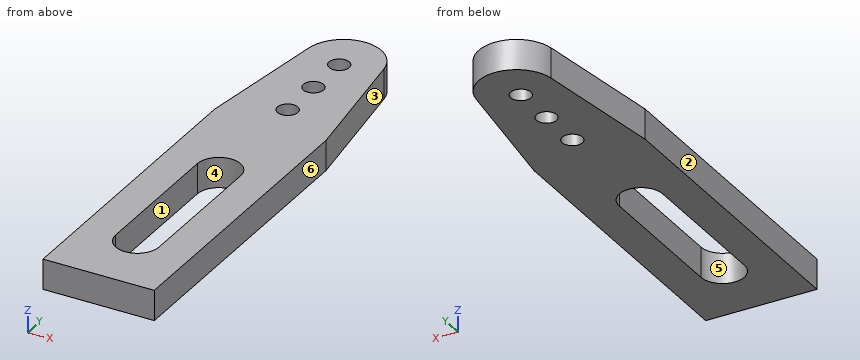
Autodesk Inventor part; units mm, degrees
ref_plane "YZ Plane" through (0, 0, 0) normal (1, 0, 0) x (0, 1, 0)
ref_plane "XZ Plane" through (0, 0, 0) normal (0, 1, 0) x (-1, 0, 0)
ref_plane "XY Plane" through (0, 0, 0) normal (0, 0, 1) x (1, 0, 0)
sketch "Sketch1" plane through (0, 0, 0) normal (0, 0, 1) x (1, 0, 0)
  line L0 (0, 0) -> (7.35, 0)
  line L1 (7.35, 0) -> (7.35, 20)
  line L2 (7.35, 20) -> (0, 20)
  line L3 (0, 20) -> (0, 0)
  circle A0 centre (3.68, 28.5) radius 2.5
  line L4 (1.2028, 28.8372) -> (0, 20)
  line L5 (6.1575, 28.8344) -> (7.35, 20)
  circle A1 centre (3.68, 28) radius 0.67
  circle A2 centre (3.68, 4.5) radius 1.43
  circle A3 centre (3.68, 14) radius 1.43
  circle A4 centre (3.68, 25) radius 0.67
  circle A5 centre (3.68, 22) radius 0.67
  line L6 (2.25, 4.5) -> (2.25, 14)
  line L7 (5.11, 14) -> (5.11, 4.5)
  point P0 (5.11, 4.5)
  dimension "d0" = 7.35
  dimension "d1" = 20
  dimension "d2" = 5
  dimension "d3" = 28.5
  dimension "d4" = 3.68
  dimension "d5" = 1.34
  dimension "d6" = 2.86
  dimension "d7" = 2.86
  dimension "d8" = 1.34
  dimension "d9" = 1.34
  dimension "d10" = 28
  dimension "d11" = 3.68
  dimension "d12" = 25
  dimension "d13" = 3.68
  dimension "d14" = 3.68
  dimension "d15" = 22
  dimension "d16" = 14
  dimension "d17" = 4.5
  dimension "d18" = 3.68
  dimension "d19" = 3.68
extrude "Extrusion1" add sketch "Sketch1" along normal blind 2
properties part number "Standard Servo Horn - Linear Arm"
Verification items for the finished model (mm, model axes). Face numbers are marked on the shaded views. A direction names the side the tool comes from. Give positions to 0.01 mm unless a question says otherwise; leave off trailing zeros. Write each loop counter-clockwise with the first axis right and the second up, starting at its lowest first coordinate (ties: lowest second). Pieces come first, ordered by that corner, then holes. Notation, with made-up numbers: M 88,43.25 L 92,43.25 A7 cw 92,50.25 Z; hole C -0.75,42 d5. An arc over 180 degrees is marked long. Write item = value, one per line.
(1) Access from +Z, -Z, +X, -X, +Y, -Y to the whole of each face (thin tool, end or side, straight path). Record for the marked faces 5 and 6.
Found:
face_5 = +Z, -Z
face_6 = +Z, -Z, +X, +Y, -Y
(2) Sectioned sample at D-D (y = 28). Record the cut outline in (x, z), then the cut area to 3 significant figures.
Found:
outline = M 1.09,0 L 3.01,0 L 3.01,2 L 1.09,2 Z; M 4.35,0 L 6.27,0 L 6.27,2 L 4.35,2 Z
area = 7.68 mm2
(3) Sectioned sample at C-C (z = 1). Record the cut outline in (x, y), then the cut area to 3 significant figures.
Found:
outline = M 0,0 L 7.35,0 L 7.35,20 L 6.16,28.83 A2.5 ccw 1.2,28.84 L 0,20 Z; hole M 2.25,4.5 A1.43 ccw 5.11,4.5 L 5.11,14 A1.43 ccw 2.25,14 Z; hole C 3.68,22 d1.34; hole C 3.68,25 d1.34; hole C 3.68,28 d1.34
area = 172 mm2
(4) Draft check along Y on the marked faces 1, 2, 3 and 4. Enter one of: released by +Y, released by -Y, zero draft, split by the parting line, or undercut.
Found:
face_1 = undercut
face_2 = zero draft
face_3 = released by +Y
face_4 = undercut
(5) Sectioned sample at B-B (x = 3.68). Record the cut outline in (y, z).
Found:
outline = M 0,0 L 3.07,0 L 3.07,2 L 0,2 Z; M 15.43,0 L 21.33,0 L 21.33,2 L 15.43,2 Z; M 22.67,0 L 24.33,0 L 24.33,2 L 22.67,2 Z; M 25.67,0 L 27.33,0 L 27.33,2 L 25.67,2 Z; M 28.67,0 L 31,0 L 31,2 L 28.67,2 Z
(6) Sectioned sample at A-A (y = 8). Record the cut outline in (x, z).
Found:
outline = M 0,0 L 2.25,0 L 2.25,2 L 0,2 Z; M 5.11,0 L 7.35,0 L 7.35,2 L 5.11,2 Z
(7) Material ranges on line 1 (Y direction, x = 3.68, z = 0.75); line 2 (X direction, y = 13, z = 1.9); line 3 (Y direction, x = 4.25, z = 1.2), recorded low to high.
Found:
line_1 = 0 to 3.07, 15.43 to 21.33, 22.67 to 24.33, 25.67 to 27.33, 28.67 to 31
line_2 = 0 to 2.25, 5.11 to 7.35
line_3 = 0 to 3.19, 15.31 to 21.65, 22.35 to 24.65, 25.35 to 27.65, 28.35 to 30.93
(8) Go/stop test with a flat-tipped pin: pin 1 Ø0.8 at (x, y) = (3.68, 22) entering from -Z. Record where the tip stops, or that it passes through.
Found:
pin_1 = through
